```python
from build123d import *

# Parameters (mm, degrees)
F0_W     = 12.7
F0_H     = 7.9375
F1_DEPTH = 1.5875


with BuildPart() as f1:
    # F0 (on Front) → F1 (new body, symmetric)
    with BuildSketch(Plane.XZ):
        Polygon((57.15, -5.794347), (-57.15, -5.794347), (-57.15, -12.144347), (-60.325, -12.144347), (-60.325, -24.844347), (-57.15, -24.844347), (-57.15, -31.194347), (-22.225, -31.194347), (-22.225, -26.352472), (-24.41575, -26.352472), (-24.41575, -23.574347), (-22.225, -23.574347), (-22.225, -18.494347), (-18.669, -18.494347), (-18.669, -23.574347), (-16.47825, -23.574347), (-16.47825, -26.352472), (-18.669, -26.352472), (-18.669, -31.194347), (18.669, -31.194347), (18.669, -26.352472), (16.47825, -26.352472), (16.47825, -23.574347), (18.669, -23.574347), (18.669, -18.494347), (22.225, -18.494347), (22.225, -23.574347), (24.41575, -23.574347), (24.41575, -26.352472), (22.225, -26.352472), (22.225, -31.194347), (57.15, -31.194347), (57.15, -24.844347), (60.325, -24.844347), (60.325, -12.144347), (57.15, -12.144347), align=None)
        with Locations((0.695352, -16.113097)):
            Rectangle(F0_W, F0_H, mode=Mode.SUBTRACT)
    extrude(amount=F1_DEPTH, both=True)


solid = f1.part
```
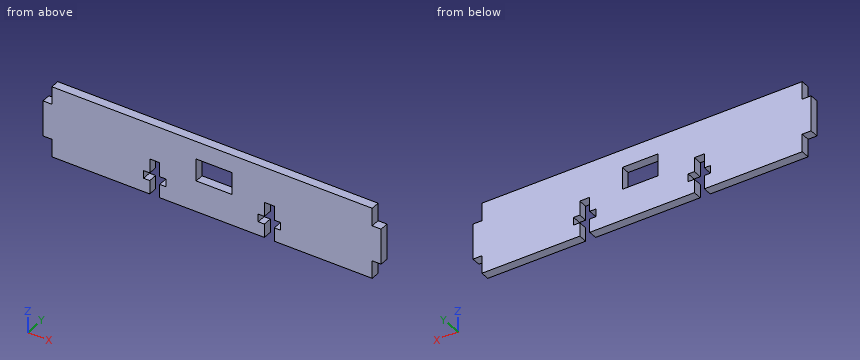
Model file for the job. Use its own axes, mm. Coordinates: 2 decimals unless noted, no trailing zeros. Write each loop counter-clockwise with the first axis right and the second up, starting at its lowest first coordinate (ties: lowest second). Pieces come first, ordered by that corner, then holes. Notation, with made-up numbers: (-6.75, 40.5) - (7.25, 40.5) arc R15 cw to (7.25, 60.5) - close; hole circle Ø11 at (36.5, 75). An arc over 180 degrees is marked (long way). One line per question, with ' | ' between items. Start each with the question number.
Q1. Cut at A-A, the plane z = -22.5. List the corners of the cut face in (x, y) (1 decimal).
Q2. Drill centre lines: line 1 (X direction, y = 1.2, z = -19.5) (3 decimals); line 2 (X direction, y = -0.75, z = -28.25) (3 decimals); line 3 (X direction, y = -0.75, z = -23) (3 decimals). Where is each one in solid material? Low to high. Write a range as [from, to].
Q3. Cut at B-B, the plane x = 1. List the corners of the cut face in (y, z), then the cut area to 3 significant figures.
Q4. Cut at D-D, the plane z = -9. List the corners of the cut face in (x, y), then the cut area to 3 significant figures.
Q5. Pin check, flat tips, straight feed: pin 1 (1.6 mm diameter, centred on x = 20, y = 0, fed in from -Z); pin 2 (1 mm diameter, centred on y = 0, z = -8.5, fed in from +X). Stop position of each tip, or through.
Q6. Cut at C-C, the plane z = -16.5. List the corners of the cut face in (x, y) (1 decimal), then the cut area to 3 significant figures.
Answer below:
1) outline: (-60.3, -1.6) - (-22.2, -1.6) - (-22.2, 1.6) - (-60.3, 1.6) - close; (-18.7, -1.6) - (18.7, -1.6) - (18.7, 1.6) - (-18.7, 1.6) - close; (22.2, -1.6) - (60.3, -1.6) - (60.3, 1.6) - (22.2, 1.6) - close
2) line 1: [-60.325, -22.225], [-18.669, -5.655], [7.045, 18.669], [22.225, 60.325] | line 2: [-57.15, -22.225], [-18.669, 18.669], [22.225, 57.15] | line 3: [-60.325, -22.225], [-18.669, 18.669], [22.225, 60.325]
3) outline: (-1.59, -31.19) - (1.59, -31.19) - (1.59, -20.08) - (-1.59, -20.08) - close; (-1.59, -12.14) - (1.59, -12.14) - (1.59, -5.79) - (-1.59, -5.79) - close | area: 55.4 mm^2
4) outline: (-57.15, -1.59) - (57.15, -1.59) - (57.15, 1.59) - (-57.15, 1.59) - close | area: 363 mm^2
5) pin 1: z = -18.49 | pin 2: x = 57.15
6) outline: (-60.3, -1.6) - (-5.7, -1.6) - (-5.7, 1.6) - (-60.3, 1.6) - close; (7, -1.6) - (60.3, -1.6) - (60.3, 1.6) - (7, 1.6) - close | area: 343 mm^2
